Autodesk Inventor part; units mm, degrees
ref_plane "YZ Plane" through (0, 0, 0) normal (1, 0, 0) x (0, 1, 0)
ref_plane "XZ Plane" through (0, 0, 0) normal (0, 1, 0) x (-1, 0, 0)
ref_plane "XY Plane" through (0, 0, 0) normal (0, 0, 1) x (1, 0, 0)
sketch "Boceto1" plane through (0, 0, 0) normal (0, 1, 0) x (-1, 0, 0)
  line L0 (20, -10) -> (20, -16)
  line L1 (50, -16) -> (50, -16.5)
  line L2 (50, -16.5) -> (49.0807, -16.5)
  circle A0 centre (0, -33) radius 1.5
  circle A1 centre (0, -33) radius 3
  arc A2 (0, -26) -> (5.7446, -37) centre (0, -33) ccw
  line L3 (5.7446, -37) -> (35, -37)
  line L4 (35, -37) -> (50, -19)
  line L5 (0, -23) -> (20, -23)
  line L6 (20, -23) -> (20, -17)
  line L7 (20, -17) -> (50, -17)
  line L8 (50, -17) -> (50, -19)
  line L9 (0, -31.5) -> (0, -30)
  line L10 (0, -26) -> (0, -23)
  point P0 (0, -37)
  dimension "d8" = 6
  dimension "d9" = 0.5
extrude "Extrusión1" add sketch "Boceto1" along normal blind 8 contours A1 | L10 L5 L6 L7 L8 L4 L3 A2
sketch "Boceto6" plane through (0, 0, 0) normal (0, -1, 0) x (1, 0, 0)
  line L0 (-50, -17) -> (-20, -17)
  line L1 (-50, -16) -> (-50, -14)
  line L2 (-50, -17) -> (-50, -16)
  line L3 (-50, -16.5) -> (-16.403, -16.5)
  line L4 (-20, -23) -> (-25, -23)
  line L5 (-5.7446, -37) -> (-35, -37)
  line L6 (-25, -23) -> (-25, -28)
  line L7 (-25, -37) -> (-25, -32)
  line L8 (-25, -32) -> (-5.7446, -32)
  line L9 (-5.7446, -32) -> (-5.7446, -27.061)
  line L10 (-25, -28) -> (-5.7446, -28)
  line L11 (-35, -37) -> (-30, -37)
  line L12 (-30, -37) -> (-30, -32)
  line L13 (-30, -32) -> (-25, -32)
  line L14 (-50, -19) -> (-50, -17)
  line L15 (-50, -19) -> (-45, -19)
  line L16 (-30, -37) -> (-45, -19)
  line L17 (-45, -19) -> (-40, -19)
  line L18 (-30, -32) -> (-40.8333, -19)
  line L19 (-40.8333, -19) -> (-25, -19)
  line L20 (-25, -19) -> (-25, -28)
  line L21 (-30, -32) -> (-34.1667, -32)
  line L22 (-40.8333, -19) -> (-35.8333, -19)
  line L23 (-35.8333, -19) -> (-25, -32)
  line L24 (-35.8333, -19) -> (-30.8333, -19)
  line L25 (-25, -32) -> (-20, -32)
  line L26 (-20, -32) -> (-30.8333, -19)
  line L27 (-30, 4) -> (-45, -14)
  line L28 (-45, -14) -> (-40, -14)
  line L29 (-30, -1) -> (-40.8333, -14)
  line L30 (-30, -1) -> (-34.1667, -1)
  line L31 (-35.8333, -14) -> (-25, -1)
  line L32 (-35.8333, -14) -> (-30.8333, -14)
  line L33 (-25, -1) -> (-20, -1)
  line L34 (-20, -1) -> (-30.8333, -14)
  point P0 (0, 0)
  dimension "d28" = 5
  dimension "d29" = 5
  dimension "d30" = 5
  dimension "d31" = 5
  dimension "d32" = 5
  dimension "d33" = 5
  dimension "d34" = 5
  dimension "d35" = 5
  dimension "d36" = 5
extrude "Extrusión6" cut sketch "Boceto6" against normal blind 10 contours L23 L19 L26 L6 L10 L8 | L21 L16 L17 L18 | L10 L6 L26 | L30 L29 L28 L27 | L31 L33 L34 L32
sketch "Boceto7" plane through (0, 0, 0) normal (0, -1, 0) x (1, 0, 0)
  line L0 (-35, 4) -> (-5.7446, 4)
  arc A0 (7, 0) -> (-5.7446, 4) centre (0, 0) ccw
  line L1 (-5.7446, 4) -> (7, 0)
  line L2 (7, 0) -> (8.04, 10.76)
  line L3 (8.04, 10.76) -> (-8.8935, 9.8507)
  line L4 (-8.8935, 9.8507) -> (-5.7446, 4)
extrude "Extrusión7" cut sketch "Boceto7" against normal blind 10 contours L1 A0
chamfer "Chaflán1" distance 2 angle 45 2 edges at (-50, 4, -19) (0, 4, -23)
sketch "Boceto9" plane through (0, 0, 0) normal (0, -1, 0) x (1, 0, 0)
  circle A0 centre (0, -33) radius 1.5
  circle A1 centre (0, -33) radius 3
  point P0 (0, 0)
  dimension "d47" = 6
extrude "Extrusión9" cut sketch "Boceto9" against normal blind 4
sketch "Boceto10" plane through (0, 8, 0) normal (0, 1, 0) x (1, 0, 0)
  circle A0 centre (0, 33) radius 1.5
  circle A1 centre (0, 33) radius 6
  line L0 (0, 33) -> (-19, 33)
  line L1 (0, 33) -> (0, 37.5)
  line L2 (0, 37.5) -> (-19, 37.5)
  line L3 (-19, 37.5) -> (-19, 28.5)
  line L4 (-19, 28.5) -> (0, 28.5)
  line L5 (-19, 33) -> (-16, 33)
  circle A2 centre (-16, 33) radius 3
  circle A3 centre (-16, 33) radius 3
  line L6 (-16, 36) -> (-3.9686, 37.5)
  line L7 (-16, 33) -> (-16, 30)
  line L8 (-16, 30) -> (-3.9686, 28.5)
  point P0 (0, 0)
  dimension "d50" = 12
  dimension "d51" = 19
  dimension "d52" = 4.5
  dimension "d53" = 9
  dimension "d54" = 3
extrude "Extrusión10" cut sketch "Boceto10" against normal blind 2 contours A0 L1 L2 A1 L0 | A0 L0 A1 L2 L1 | L0 A2 L6 A1 | A1 L8 A2 L0 | A2 L7 L0 | L0 A2 | A2 L0 L7
properties part number "pinza dcha sg996r"
Here's how the part is built. I have some questions about the finished solid (model axes, mm). A direction names the side the tool comes from. Coordinates: 2 decimals unless noted, no trailing zeros. Loops run counter-clockwise (first coordinate to the right, second up) from the corner with the lowest first, then second, coordinate; pieces in that order, holes last.
1. If we mould it in two halves opening along X, with no side actions, what happens to faces 1 (the flat face through (1.3, 4, -34.3)), 2 (the flat face through (-41.764, 3.944, -28.883)), 3 (the flat face through (-1, 4, -24)), 4 (the flat face through (-21, 0, -28))? For each: pulls with the +X half, pulls with the -X half, needs draft (parallel to the pull), parting line crosses it, or undercut.
2. Imagine slicing it at A-A, the plane y = 2.75. Count the separate pieces of the cut face and the enclosed holes in it, and give its area (3 significant figures).
3. For faces 5 (the flat face through (-23, 4, -32)), 6 (the cylindrical face through (-0.65, 1.97, -35.93)), 7 (the flat face through (-4.754, 7.014, -37.402)), 8 (the flat face through (-20, 4, -37)), 9 (the flat face through (-20, 4, -20)), which set-ups out of +Z, -Z, +X, -X, +Y, -Y let a thin tool reach every point of the face, with its end or its side?
4. Imagine slicing it at D-D, the plane x = -15. Please give me the cut outline in (y, z), and give its area (3 significant figures).
5. I need wall thicknesses on L1, parallel to Y at x = -10.5, z = -34.25; L2, parallel to X at y = 0.75, z = -21.75; L3, parallel to X at y = 5.05, z = -33. Which ranges of each line are inside material? Lowest first, please.
6. Imagine slicing it at C-C, the plane z = -33. Please give me the cut outline in (x, y).
7. For P1, Ø2, axis at y = 2, z = -31, coming from the -X side; P2, Ø1.3, axis at x = -42.5, y = 5, coming from the -Z side; P3, Ø1.5, axis at x = -38, z = -22.5, coming from the +Y side; P4, Ø1, axis at y = 6, z = -21, coming from the +X side, each with a flat end and sliding along its axis, tell me the tip position at first contact or that it passes through.
8. Imagine slicing it at B-B, the plane z = -23.5. Please give me the cut outline in (x, y).
Taken from the geometry:
1. face 1: undercut
1. face 2: pulls with the -X half
1. face 3: pulls with the +X half
1. face 4: needs draft
2. separate pieces: 1
2. enclosed holes: 3
2. area: 683 mm2
3. face 5: +Y, -Y
3. face 6: -Y
3. face 7: +Y
3. face 8: -Z, -X, +Y, -Y
3. face 9: +Z, +X, +Y, -Y
4. outline: (0, -37) - (8, -37) - (8, -36.12) - (6, -36.12) - (6, -29.88) - (8, -29.88) - (8, -23) - (0, -23) - close
4. area: 99.5 mm2
5. L1: y = 0 to 6
5. L2: x = -47.71 to -42.71, -38.54 to -33.54, -28.54 to -20
5. L3: x = -38.33 to -1.5, 1.5 to 7
6. outline: (-38.33, 0) - (-3, 0) - (-3, 4) - (-1.5, 4) - (-1.5, 6) - (-19, 6) - (-19, 8) - (-38.33, 8) - close; (1.5, 4) - (3, 4) - (3, 0) - (7, 0) - (7, 8) - (6, 8) - (6, 6) - (1.5, 6) - close
7. P1: stops at x = -40.83
7. P2: stops at z = -28.78
7. P3: stops at y = 8
7. P4: stops at x = -20
8. outline: (-46.25, 0) - (-41.25, 0) - (-41.25, 8) - (-46.25, 8) - close; (-37.08, 0) - (-32.08, 0) - (-32.08, 8) - (-37.08, 8) - close; (-27.08, 0) - (-1.5, 0) - (-1.5, 8) - (-27.08, 8) - close
